Check sheet for the drawn part. Datum: minimum x, y, z corner. Units: mm. A direction names the side the tool comes from. Coordinates: 2 decimals unless noted, no trailing zeros. Order: outer loops, then holes, each group sorted by start corner. A loop starts at its lowest first (then second) coordinate and runs counter-clockwise, first axis right, second up. Notation, with made-up numbers: (76, -36) - (119, -36) arc R13 ccw to (119, -32) - close; hole circle Ø2 at (1, 41.25). An arc over 180 degrees is marked (long way). Put each result on its own line as item: value.
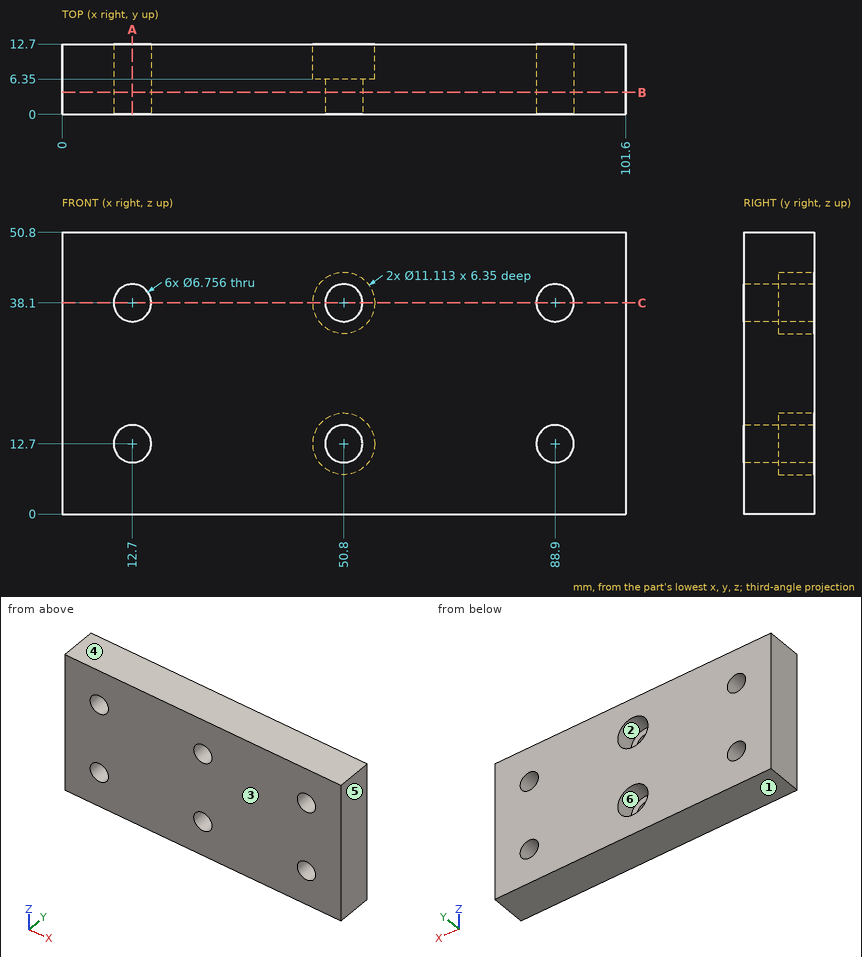
Q1. Section check A-A on x = 12.7. Record the boundary of the cut face in (y, z).
Answer block:
outline: (0, 0) - (12.7, 0) - (12.7, 9.32) - (0, 9.32) - close; (0, 16.08) - (12.7, 16.08) - (12.7, 34.72) - (0, 34.72) - close; (0, 41.48) - (12.7, 41.48) - (12.7, 50.8) - (0, 50.8) - close
Q2. Section check C-C on z = 38.1. Record the boundary of the cut face in (x, y).
Answer block:
outline: (0, 0) - (9.32, 0) - (9.32, 12.7) - (0, 12.7) - close; (16.08, 0) - (47.42, 0) - (47.42, 6.35) - (45.24, 6.35) - (45.24, 12.7) - (16.08, 12.7) - close; (54.18, 0) - (85.52, 0) - (85.52, 12.7) - (56.36, 12.7) - (56.36, 6.35) - (54.18, 6.35) - close; (92.28, 0) - (101.6, 0) - (101.6, 12.7) - (92.28, 12.7) - close
Q3. Access from +Z, -Z, +X, -X, +Y, -Y to the whole of each face (thin tool, end or side, straight path). Record for the marked faces 5 and 6.
Answer block:
face 5: +Z, -Z, +X, +Y, -Y
face 6: +Y
Q4. Draft check along Z on the marked faces 1, 2, 3 and 4. Enter one of: pulls with the +Z half, pulls with the -Z half, needs draft (parallel to the pull), parting line crosses it, or undercut.
Answer block:
face 1: pulls with the -Z half
face 2: undercut
face 3: needs draft
face 4: pulls with the +Z half
Q5. Depth check by flat-ended pin: pin 1 Ø3.5 at (x, z) = (48.5, 35.5) entering from +Y. Enter the tip coordinate at first touch or a pass-through.
Answer block:
pin 1: stops at y = 6.35
Q6. Section check B-B on y = 4. Record the boundary of the cut face in (x, z), then the cut area to 3 significant figures.
Answer block:
outline: (0, 0) - (101.6, 0) - (101.6, 50.8) - (0, 50.8) - close; hole circle Ø6.76 at (12.7, 12.7); hole circle Ø6.76 at (12.7, 38.1); hole circle Ø6.76 at (50.8, 12.7); hole circle Ø6.76 at (50.8, 38.1); hole circle Ø6.76 at (88.9, 12.7); hole circle Ø6.76 at (88.9, 38.1)
area: 4,950 mm^2
Q7. Thickness scan on L1, parallel to Z at x = 50.8, y = 5; L2, parallel to X at y = 6.75, z = 12.5; L3, parallel to Z at x = 50.8, y = 8.25. Record the ranges inside material, lowest first. Write a range as [from, to].
Answer block:
L1: z = [0, 9.32], [16.08, 34.72], [41.48, 50.8]
L2: x = [0, 9.33], [16.07, 45.25], [56.35, 85.53], [92.27, 101.6]
L3: z = [0, 7.14], [18.26, 32.54], [43.66, 50.8]
